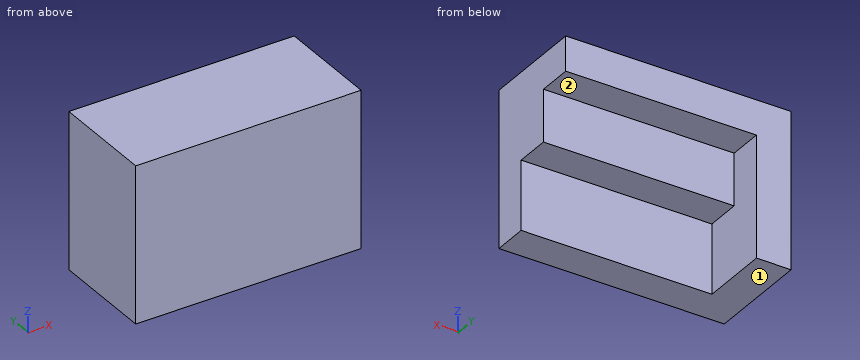
from build123d import *

# Parameters (mm, degrees)
SKETCH1_W           = 104
SKETCH1_H           = 72
BOSS_EXTRUDE1_DEPTH = 16
SKETCH3_W           = 16
SKETCH3_H           = 48
BOSS_EXTRUDE2_DEPTH = 104
SKETCH6_W           = 16
SKETCH6_H           = 48
BOSS_EXTRUDE3_DEPTH = 72
SKETCH7_W           = 88
SKETCH7_H           = 24
BOSS_EXTRUDE4_DEPTH = 16


with BuildPart() as part:
    # Sketch1 → Boss-Extrude1 (new body)
    with BuildSketch(Plane(origin=(0, 0, 0), x_dir=(1, 0, 0), z_dir=(0, 1, 0))):
        with Locations((52, 36)):
            Rectangle(SKETCH1_W, SKETCH1_H)
    extrude(amount=BOSS_EXTRUDE1_DEPTH)

    # Sketch3 → Boss-Extrude2 (add)
    with BuildSketch(Plane.ZY):
        with Locations((-8, 24)):
            Rectangle(SKETCH3_W, SKETCH3_H)
    extrude(amount=-BOSS_EXTRUDE2_DEPTH)

    # Sketch6 → Boss-Extrude3 (add)
    with BuildSketch(Plane(origin=(0, 0, -72), x_dir=(-1, 0, 0), z_dir=(0, 0, -1))):
        with Locations((-8, 24)):
            Rectangle(SKETCH6_W, SKETCH6_H)
    extrude(amount=-BOSS_EXTRUDE3_DEPTH)

    # Sketch7 → Boss-Extrude4 (add)
    with BuildSketch(Plane(origin=(0, 16, 0), x_dir=(1, 0, 0), z_dir=(0, 1, 0))):
        with Locations((60, 28)):
            Rectangle(SKETCH7_W, SKETCH7_H)
    extrude(amount=BOSS_EXTRUDE4_DEPTH)


solid = part.part
Can you work these out from the model? Positions are in its coordinate system, mm. Face numbers are marked on the shaded views. A direction names the side the tool comes from. Give positions to 0.01 mm unless a question says otherwise; leave off trailing zeros. Order: outer loops, then holes, each group sorted by start corner. A loop starts at its lowest first (then second) coordinate and runs counter-clockwise, first axis right, second up. Notation, with made-up numbers: M 13.25,20.25 L 26.25,20.25 A29 cw 26.25,56.25 Z; hole C 82,45.5 d4. An arc over 180 degrees is marked long. Use a Markdown table: item, result. Add a question column.
Item 1: Suppose I cut it at C-C (y = 20). List the corners of the cut face in (x, z) for me.
Item 2: Will these pins go through, and if not, where does the flat tip stop? pin 1 (4 mm diameter, centred on x = 19, y = 34.5, fed in from -Z); pin 2 (3 mm diameter, centred on y = 21.5, z = -47, fed in from +X); pin 3 (7 mm diameter, centred on x = 78.5, z = -24, fed in from +Y).
Item 3: Suppose I cut it at A-A (x = 59). List the corners of the cut face in (y, z) for me.
Item 4: Suppose I cut it at B-B (z = -37.5). List the corners of the cut face in (x, y) for me.
Item 5: For the marked faces 1 and 2, which set-ups out of +Z, -Z, +X, -X, +Y, -Y let a thin tool reach every point of the face, with its end or its side?
Item 6: If I drill on L1, parallel to Y at x = 74.5, z = -31; L2, parallel to Y at x = 21.5, z = -55.5; L3, parallel to Z at x = 49.5, y = 31.5, over which ranges is the centre line in solid material (lowest first)? Write a range as [from, to].
Answer sheet:
| question | item | result |
|---|---|---|
| 1 | outline | M 0,-72 L 16,-72 L 16,-40 L 104,-40 L 104,0 L 0,0 Z |
| 2 | pin 1 | stops at z = -16 |
| 2 | pin 2 | stops at x = 16 |
| 2 | pin 3 | stops at y = 32 |
| 3 | outline | M 0,-72 L 16,-72 L 16,-40 L 32,-40 L 32,-16 L 48,-16 L 48,0 L 0,0 Z |
| 4 | outline | M 0,0 L 104,0 L 104,32 L 16,32 L 16,48 L 0,48 Z |
| 5 | face 1 | -Z, +X, -X, +Y, -Y |
| 5 | face 2 | -Z, +X, +Y |
| 6 | L1 | y = [0, 32] |
| 6 | L2 | y = [0, 16] |
| 6 | L3 | z = [-40, 0] |
